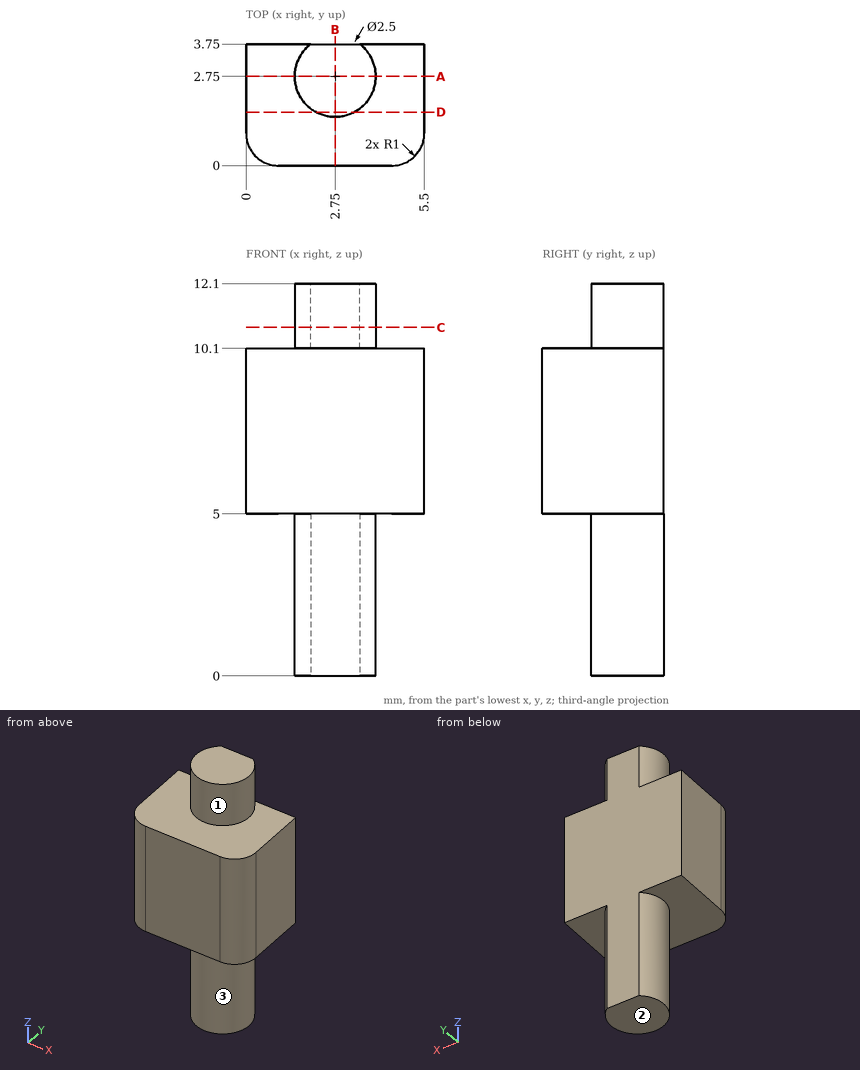
Geometry check sheet. Reference: drawing and pictorial views, mm from the part's lowest x, y, z. A direction names the side the tool comes from. Coordinates: 2 decimals unless noted, no trailing zeros. Order: outer loops, then holes, each group sorted by start corner. A loop starts at its lowest first (then second) coordinate and runs counter-clockwise, first axis right, second up.
1. Sectioned sample at D-D, the plane y = 1.65. Record the cut outline in (x, z).
Results found:
outline: (0, 5) - (2.16, 5) - (2.16, 0) - (3.34, 0) - (3.34, 5) - (5.5, 5) - (5.5, 10.1) - (3.34, 10.1) - (3.34, 12.1) - (2.16, 12.1) - (2.16, 10.1) - (0, 10.1) - close
2. Scan lines: line 1 (Z direction, x = 2.15, y = 0.5); line 2 (X direction, y = 3.2, z = 1.75); line 3 (X direction, y = 1.75, z = 3). Record each from-to range of solid material in increasing order.
Results found:
line 1: z = 5 to 10.1
line 2: x = 1.58 to 3.92
line 3: x = 2 to 3.5
3. Sectioned sample at B-B, the plane x = 2.75. Record the cut outline in (y, z), and give its area (3 significant figures).
Results found:
outline: (0, 5) - (1.5, 5) - (1.5, 0) - (3.75, 0) - (3.75, 12.1) - (1.5, 12.1) - (1.5, 10.1) - (0, 10.1) - close
area: 34.9 mm2
4. Set-up check for the marked faces 1, 2 and 3: record each of +Z, -Z, +X, -X, +Y, -Y from which the full face is reachable in a straight line by a thin tool's end or side.
Results found:
face 1: +Z
face 2: -Z, +X, -X, +Y, -Y
face 3: -Z
5. Sectioned sample at C-C, the plane z = 10.75. Record the cut outline in (x, y).
Results found:
outline: (2, 3.75) arc R1.25 ccw (long way) to (3.5, 3.75) - close
6. Sectioned sample at A-A, the plane y = 2.75. Record the cut outline in (x, z).
Results found:
outline: (0, 5) - (1.5, 5) - (1.5, 0) - (4, 0) - (4, 5) - (5.5, 5) - (5.5, 10.1) - (4, 10.1) - (4, 12.1) - (1.5, 12.1) - (1.5, 10.1) - (0, 10.1) - close
